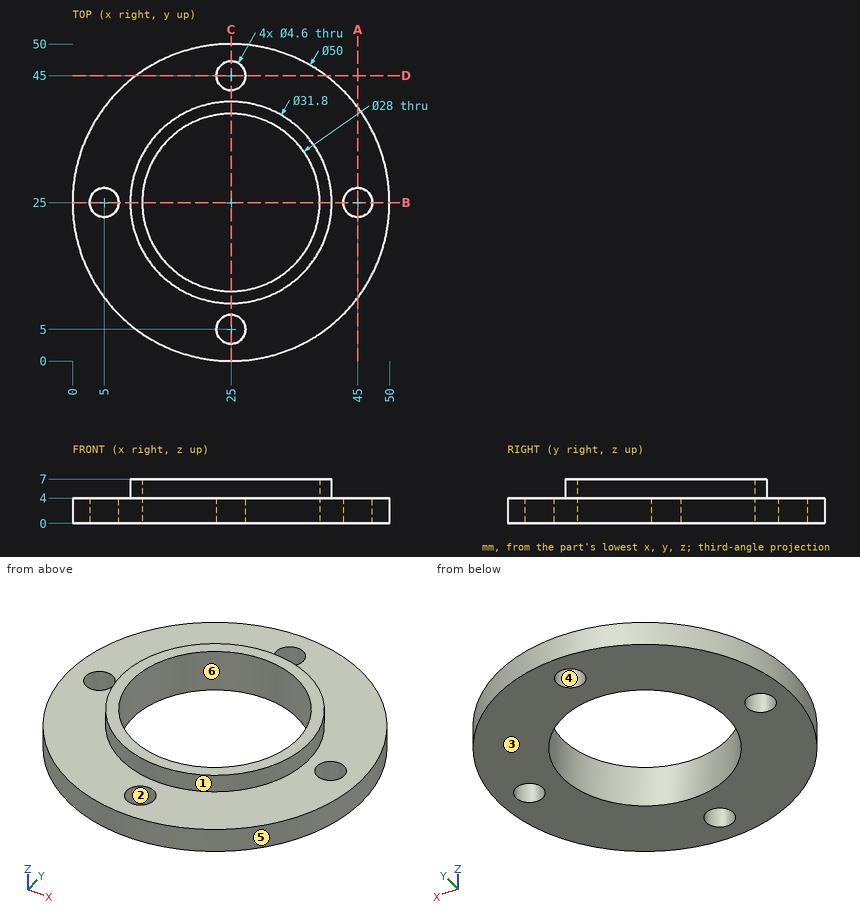
For this review, use the dimensioned drawing (mm, ordinates from the lowest corner) and the shaded views. A direction names the side the tool comes from. Round coordinates to 2 decimals unless told otherwise and drop trailing zeros. Write each loop counter-clockwise with the first axis right and the second up, starting at its lowest first coordinate (ties: lowest second). Pieces come first, ordered by that corner, then holes. Notation, with made-up numbers: (3, 62) -> (42, 62) arc R13 cw to (42, 81) -> close; hole circle Ø7 at (36.5, -36.75). An arc over 180 degrees is marked (long way). Use CSV: the item, a comma, the result in double quotes.
(1) Clearance check with flat-ended pins moving along their axes: P1, Ø7.5, axis at x = 25, y = 45, coming from the -Z side; P2, Ø3.5, axis at x = 5, y = 25, coming from the -Z side; P3, Ø3, axis at y = 35, z = 6, coming from the +X side; P4, Ø1, axis at y = 41, z = 1.5, coming from the +X side. State where each tip first meets the part, or that it passes through.
Computed values:
P1,"z = 0"
P2,"through"
P3,"x = 38.44"
P4,"x = 44.62"
(2) Draft analysis for pull direction X (two halves, no side actions). For the marked faces 3, 4, 5 and 6, state which applies: +X half, -X half, draft (parallel to the pull), parting line (faces both ways), or undercut.
Computed values:
face 3,"draft"
face 4,"undercut"
face 5,"parting line"
face 6,"undercut"
(3) Consider section B-B, the plane y = 25. Give the boundary of the cut face in (x, z).
Computed values:
outline,"(0, 0) -> (2.7, 0) -> (2.7, 4) -> (0, 4) -> close; (7.3, 0) -> (11, 0) -> (11, 7) -> (9.1, 7) -> (9.1, 4) -> (7.3, 4) -> close; (39, 0) -> (42.7, 0) -> (42.7, 4) -> (40.9, 4) -> (40.9, 7) -> (39, 7) -> close; (47.3, 0) -> (50, 0) -> (50, 4) -> (47.3, 4) -> close"
(4) To check wall thickness, follow L1, parallel to X at y = 28, z = 1.75; L2, parallel to Y at x = 34, z = 2.25; L3, parallel to X at y = 7, z = 1.75. State the ranges of each line that lie inside material, in increasing order. Write a range as [from, to].
Computed values:
L1,"[0.18, 11.33], [38.67, 49.82]"
L2,"[1.68, 14.28], [35.72, 48.32]"
L3,"[7.65, 23.86], [26.14, 42.35]"
(5) For the marked faces 1 and 2, list the 3-axis set-ups (+Z, -Z, +X, -X, +Y, -Y) from which the entire face can be reached by the end or side of a thin tool; tool diameter is ignored.
Computed values:
face 1,"+Z"
face 2,"+Z, -Z"
(6) Consider section A-A, the plane x = 45. Give the boundary of the cut face in (y, z), plus the area to 3 significant figures.
Computed values:
outline,"(10, 0) -> (22.7, 0) -> (22.7, 4) -> (10, 4) -> close; (27.3, 0) -> (40, 0) -> (40, 4) -> (27.3, 4) -> close"
area,"102 mm²"
